Can you work these out from the model? Positions are in its coordinate system, mm. Face numbers are marked on the shaded views. A direction names the side the tool comes from. Coordinates: 2 decimals unless noted, no trailing zeros. Order: outer loops, then holes, each group sorted by start corner. A loop starts at its lowest first (then second) coordinate and runs counter-clockwise, first axis right, second up. Notation, with made-up numbers: (61.25, 14) -> (68.25, 14) arc R19 cw to (68.25, 38) -> close; hole circle Ø3 at (22.5, -11). An arc over 180 degrees is marked (long way). Answer as a JSON object with one key per item and string values. Group by question number.
(1) I want a section at C-C, the plane x = 0.05. List the corners of the cut face in (y, z) for me, plus the area to 3 significant figures.
(2) For pin 1 (0.9 mm diameter, centred on x = -2.5, y = -0.5, fed in from +Z); pin 2 (0.5 mm diameter, centred on x = 2.5, y = 0.5, fed in from -Z); pin 3 (0.9 mm diameter, centred on x = -2.5, y = 0, fed in from -Z), each with a flat end and sliding along its axis, tell me the tip position at first contact or that it passes through.
(3) If we mould it in two halves opening along X, with no side actions, what happens to the marked faces 1, 2 and 3? For each: pulls with the +X half, pulls with the -X half, needs draft (parallel to the pull), parting line crosses it, or undercut.
(4) I want a section at D-D, the plane z = -0.25. List the corners of the cut face in (x, y) for me.
(5) I want a section at B-B, the plane z = -4. List the corners of the cut face in (x, y) for me.
(6) Which directions (+Z, -Z, +X, -X, +Y, -Y) give clear straight access to the entire face, cutting with the end or side of a thin tool? Please do the marked faces 4, 5, 6 and 7.
(7) I want a section at A-A, the plane z = 2.75. List the corners of the cut face in (x, y) for me, plus the area to 3 significant figures.
(8) I need wall thicknesses on line 1 (X direction, y = 0.3, z = -1); line 2 (X direction, y = -0.25, z = -4.25); line 3 (X direction, y = -0.9, z = -0.5). Which ranges of each line are inside material? Lowest first, please.
Autodesk Fusion 360 part; units mm, degrees
sketch "Sketch1" plane through (0, 0, 0) normal (0, 1, 0) x (1, 0, 0)
  line L0 (3, 0) -> (3, -0.75)
  line L1 (3, -0.75) -> (2.45, -0.75)
  line L2 (2.45, -0.75) -> (2.45, -3.75)
  line L3 (2.45, -3.75) -> (2.75, -4.1489)
  line L4 (2.75, -4.1489) -> (2, -5.75)
  line L5 (2, -5.75) -> (0, -5.75)
  line L6 (3, 0) -> (0, 0) construction
  line L7 (2.75, 4.1489) -> (2, 5.75)
  line L8 (3, 0) -> (3, 0.75)
  line L9 (2.45, 0.75) -> (2.45, 3.75)
  line L10 (2.45, 3.75) -> (2.75, 4.1489)
  line L11 (2, 5.75) -> (0, 5.75)
  line L12 (0, 0) -> (0, 6.5) construction
  line L13 (3, 0.75) -> (2.45, 0.75)
  line L14 (0, -5.75) -> (0, 5.75)
  dimension "d1" = 3
  dimension "d2" = 0.75
  dimension "d3" = 3
  dimension "d4" = 5
  dimension "d6" = 2
  dimension "d7" = 2.75
  dimension "d8" = 2.45
  dimension "d9" = 2
revolve "Revolve2" add sketch "Sketch1" angle 360 about axis through (0, 0, 5.75) along (0, 0, -1)
sketch "Sketch3" plane through (0, 0, 5.75) normal (0, 0, 1) x (-1, 0, 0)
  circle A0 centre (0, 0) radius 2
  line L0 (-5, -1.5) -> (5, -1.5)
  line L1 (5, -1.5) -> (5, 1.5)
  line L2 (5, 1.5) -> (-5, 1.5)
  line L3 (-5, 1.5) -> (-5, -1.5)
  line L4 (-5, -1.5) -> (5, 1.5) construction
  line L5 (5, -1.5) -> (-5, 1.5) construction
  line L6 (5.6117, 3.0022) -> (-6, 3.0022)
  line L7 (-6, 3.0022) -> (-6, -3)
  line L8 (-6, -3) -> (5.6117, -3)
  line L9 (5.6117, -3) -> (5.6117, 3.0022)
  circle A1 centre (0, 0) radius 2
  dimension "d12" = 10
  dimension "d13" = 3
extrude "Extrude3" cut sketch "Sketch3" against normal blind 14 contours A0 L2 A1 | A0 L0 A1 | L6 L7 L8 L9
sketch "Sketch4" plane through (0, -1.5, 0) normal (0, -1, 0) x (1, 0, 0)
  spline S0 degree 2 poles (-2.3049, 4.1489) (-1.7364, 5.1662) (-1.3229, 5.75) knots 0 0 0 0.187886 0.187886 0.187886 weights 1 1.022081 1
  spline S1 degree 2 poles (-1.9371, 3.75) (-2.1104, 3.9322) (-2.3049, 4.1489) knots 0 0 0 0.054258 0.054258 0.054258 weights 1 1.00251 1
  line L0 (-1.9371, 3.75) -> (-1.9371, 0.75)
  line L1 (-1.9371, 0.75) -> (-2.5981, 0.75)
  line L2 (-2.5981, 0.75) -> (-2.5981, -0.75)
  line L3 (-2.5981, -0.75) -> (-1.9371, -0.75)
  line L4 (-1.9371, -0.75) -> (-1.9371, -3.75)
  spline S2 degree 2 poles (-2.3049, -4.1489) (-2.1104, -3.9322) (-1.9371, -3.75) knots 0 0 0 0.054258 0.054258 0.054258 weights 1 1.00251 1
  spline S3 degree 2 poles (-1.3229, -5.75) (-1.7364, -5.1662) (-2.3049, -4.1489) knots 0 0 0 0.187886 0.187886 0.187886 weights 1 1.022081 1
  line L5 (-1.3229, -5.75) -> (1.3229, -5.75)
  spline S4 degree 2 poles (2.3049, -4.1489) (1.7364, -5.1662) (1.3229, -5.75) knots 0 0 0 0.187886 0.187886 0.187886 weights 1 1.022081 1
  spline S5 degree 2 poles (1.9371, -3.75) (2.1104, -3.9322) (2.3049, -4.1489) knots 0 0 0 0.054258 0.054258 0.054258 weights 1 1.00251 1
  line L6 (1.9371, -3.75) -> (1.9371, -0.75)
  line L7 (1.9371, -0.75) -> (2.5981, -0.75)
  line L8 (2.5981, -0.75) -> (2.5981, 0.75)
  line L9 (2.5981, 0.75) -> (1.9371, 0.75)
  line L10 (1.9371, 0.75) -> (1.9371, 3.75)
  spline S6 degree 2 poles (2.3049, 4.1489) (2.1104, 3.9322) (1.9371, 3.75) knots 0 0 0 0.054258 0.054258 0.054258 weights 1 1.00251 1
  spline S7 degree 2 poles (1.3229, 5.75) (1.7364, 5.1662) (2.3049, 4.1489) knots 0 0 0 0.187886 0.187886 0.187886 weights 1 1.022081 1
  line L11 (1.3229, 5.75) -> (-1.3229, 5.75)
  circle A0 centre (0, 0) radius 1.5 construction
  line L12 (-0.5432, 5.75) -> (-0.5, 1.4958)
  line L13 (2, 5.75) -> (0, 5.75)
  line L14 (1, 5.75) -> (1, 1.5034)
  line L15 (2, -5.75) -> (0, -5.75)
  line L16 (-0.75, -1.4919) -> (-0.7961, -5.75)
  arc A1 (0.7487, -1.4562) -> (-0.75, -1.4919) centre (0, -1.5) ccw
  line L17 (-0.7961, -5.75) -> (-0.7961, -6.4979)
  line L18 (-0.7961, -6.4979) -> (0.7464, -6.5067)
  line L19 (-0.5432, 5.75) -> (-0.5402, 6.4921)
  line L20 (-0.5402, 6.4921) -> (1, 6.5078)
  line L21 (1, 5.75) -> (1, 6.5078)
  arc A2 (-0.5, 1.4958) -> (1, 1.5034) centre (0.25, 1.5034) ccw
  spline S8 degree 2 poles (-2.3049, 4.1489) (-1.7364, 5.1662) (-1.3229, 5.75) knots 0 0 0 0.187886 0.187886 0.187886 weights 1 1.022081 1
  spline S9 degree 2 poles (-1.9371, 3.75) (-2.1104, 3.9322) (-2.3049, 4.1489) knots 0 0 0 0.054258 0.054258 0.054258 weights 1 1.00251 1
  line L22 (-1.9371, 3.75) -> (-1.9371, 0.75)
  line L23 (-1.9371, 0.75) -> (-2.5981, 0.75)
  line L24 (-2.5981, 0.75) -> (-2.5981, -0.75)
  line L25 (-2.5981, -0.75) -> (-1.9371, -0.75)
  line L26 (-1.9371, -0.75) -> (-1.9371, -3.75)
  spline S10 degree 2 poles (-2.3049, -4.1489) (-2.1104, -3.9322) (-1.9371, -3.75) knots 0 0 0 0.054258 0.054258 0.054258 weights 1 1.00251 1
  spline S11 degree 2 poles (-1.3229, -5.75) (-1.7364, -5.1662) (-2.3049, -4.1489) knots 0 0 0 0.187886 0.187886 0.187886 weights 1 1.022081 1
  line L27 (-1.3229, -5.75) -> (1.3229, -5.75)
  spline S12 degree 2 poles (2.3049, -4.1489) (1.7364, -5.1662) (1.3229, -5.75) knots 0 0 0 0.187886 0.187886 0.187886 weights 1 1.022081 1
  spline S13 degree 2 poles (1.9371, -3.75) (2.1104, -3.9322) (2.3049, -4.1489) knots 0 0 0 0.054258 0.054258 0.054258 weights 1 1.00251 1
  line L28 (1.9371, -3.75) -> (1.9371, -0.75)
  line L29 (1.9371, -0.75) -> (2.5981, -0.75)
  line L30 (2.5981, -0.75) -> (2.5981, 0.75)
  line L31 (2.5981, 0.75) -> (1.9371, 0.75)
  line L32 (1.9371, 0.75) -> (1.9371, 3.75)
  spline S14 degree 2 poles (2.3049, 4.1489) (2.1104, 3.9322) (1.9371, 3.75) knots 0 0 0 0.054258 0.054258 0.054258 weights 1 1.00251 1
  spline S15 degree 2 poles (1.3229, 5.75) (1.7364, 5.1662) (2.3049, 4.1489) knots 0 0 0 0.187886 0.187886 0.187886 weights 1 1.022081 1
  line L33 (1.3229, 5.75) -> (-1.3229, 5.75)
  line L34 (0.7487, -1.4562) -> (0.7464, -6.5067)
  dimension "d16" = 3
  dimension "d17" = 1.5
  dimension "d18" = 1.5
extrude "Extrude4" cut sketch "Sketch4" against normal blind 6 contours L11 L13 L19 L20 L21 L33 | L11 L12 L13 L14 A2 L33 | L5 L15 L16 A1 L27 L34 | L5 L15 L17 L18 L27 L34
equation "d2 = 0.8 mm - 0.05 mm"
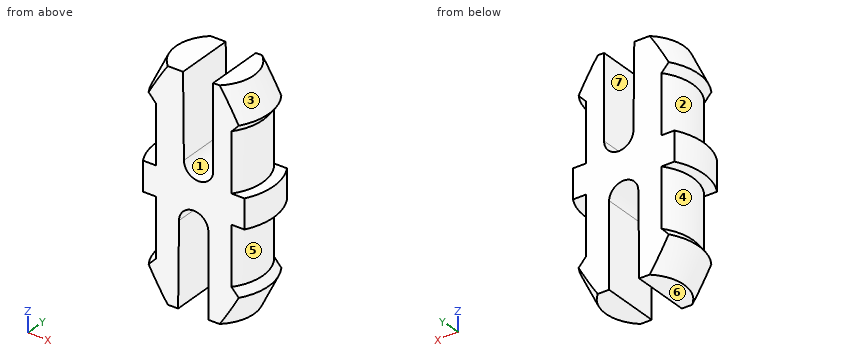
Computed values:
{
 "1": {"outline": "(-1.5, -0.75) -> (1.5, -0.75) -> (1.5, 0.78) -> (-1.5, 0.78) -> close", "area": "4.60 mm2"},
 "2": {"pin 1": "stops at z = 5.54", "pin 2": "stops at z = -5.11", "pin 3": "stops at z = -5.64"},
 "3": {"face 1": "undercut", "face 2": "pulls with the -X half", "face 3": "pulls with the +X half"},
 "4": {"outline": "(-2.6, -1.5) -> (2.6, -1.5) arc R3 ccw to (2.6, 1.5) -> (-2.6, 1.5) arc R3 ccw to start"},
 "5": {"outline": "(-2.17, -1.5) -> (-0.78, -1.5) -> (-0.78, 1.5) -> (-2.17, 1.5) arc R2.64 ccw to start; (0.75, -1.5) -> (2.17, -1.5) arc R2.64 ccw to (2.17, 1.5) -> (0.75, 1.5) -> close"},
 "6": {"face 4": "-X", "face 5": "+X", "face 6": "-Z, +X, -X, +Y, -Y", "face 7": "+Z, +Y, -Y"},
 "7": {"outline": "(-1.94, -1.5) -> (-0.51, -1.5) -> (-0.51, 1.5) -> (-1.94, 1.5) arc R2.45 ccw to start; (1, -1.5) -> (1.94, -1.5) arc R2.45 ccw to (1.94, 1.5) -> (1, 1.5) -> close", "area": "9.18 mm2"},
 "8": {"line 1": "x = -2.43 to -0.56, 0.56 to 2.43", "line 2": "x = -2.69 to -0.78, 0.75 to 2.69", "line 3": "x = -2.86 to 2.86"}
}
